Can you work these out from the model? Positions are in its coordinate system, mm. A direction names the side the tool comes from. Give positions to 0.01 mm unless a question says otherwise; leave off trailing zeros. Loops run counter-clockwise (first coordinate to the right, second up) from the corner with the lowest first, then second, coordinate; pieces in that order, holes last. Notation, with made-up numbers: (-15, 69) - (5, 69) arc R30 ccw to (5, 108) - close; hole circle Ø3 at (21.5, 85.25). An arc over 180 degrees is marked (long way). Answer as a JSON object with one key per item and string values. Group by question number.
Item 1: Suppose I cut it at B-B on z = -644.5. Write out the boundary of the cut face in (x, y).
Item 2: Thinking about a two-plate mould opening in Z: for faces 4 (the flat face through (646, 61, -711.2)), 5 (the flat face through (-650, 147, -685.8)), 6 (the flat face through (646, 132, -685.8)), 7 (the flat face through (646, -196.151, -698)), which applies, pulls with the +Z half, pulls with the -Z half, needs draft (parallel to the pull), parting line crosses it, or undercut?
Item 3: Suppose I cut it at A-A on y = 291. Write out the boundary of the cut face in (x, z).
Item 4: Please list where these lines run through material, in increasing order: L1, parallel to Y at x = 130.5, z = -12; L2, parallel to Z at x = -587, y = -171.5; L3, parallel to X at y = -108, z = -228.5.
Item 5: Which directions (+Z, -Z, +X, -X, +Y, -Y) give clear straight access to the entire face, cutting with the end or side of a thin tool? Please do faces 1 (the flat face through (646, -158, -685.8)), 2 (the flat face through (-650, -28.704, -357)), 3 (the flat face through (-650, 326.896, -698)).
Item 6: Will these pins go through, and if not, where does the flat tip stop? pin 1 (15 mm diameter, centred on x = -637, z = -520, fed in from +Y); pin 2 (2 mm diameter, centred on x = -191.5, z = -274.5, fed in from +Y); pin 3 (12.5 mm diameter, centred on x = -640.5, z = -697.5, fed in from -Y).
Item 7: Suppose I cut it at C-C on x = -510.5. Write out the boundary of the cut face in (y, z).
Item 8: Suppose I cut it at D-D on y = 100.5. Write out the boundary of the cut face in (x, z), and give its area (3 significant figures).
from build123d import *

# Parameters (mm, degrees)
F0_W           = 1346.2
F0_H           = 685.8
F1_DEPTH       = 25.4
F4_DEPTH       = 38.1
F2_W           = 50.8
F2_H           = 76.2
F5_DEPTH       = 685.8
F7_W           = 50.8
F7_H           = 25.4
F8_DEPTH       = 76.2
F8_DEPTH_BACK  = 431.8
F9_W           = 1244.6
F9_H           = 304.8
F10_DEPTH      = 25.4
F6_W           = 50.8
F6_H           = 25.4
F11_DEPTH      = 431.8
F11_DEPTH_BACK = 76.2


with BuildPart() as f1:
    # F0 (on Top) → F1 (new body)
    with BuildSketch(Plane.XY):
        with Locations((-1.6667507589, -3.4339692544)):
            Rectangle(F0_W, F0_H)
    extrude(amount=F1_DEPTH)

    # F3 (on face) → F4 (join)
    with BuildSketch(Plane(origin=(0, 0, 0), x_dir=(1, 0, 0), z_dir=(0, 0, -1))):
        Polygon((-674.7667507589, -254.2923092842), (671.4332492411, -254.2923092842), (671.4332492411, 35.8601883054), (-623.9667507589, 35.8601883054), (-623.9667507589, 28.7036430091), (-674.7667507589, 28.7036430091), align=None)
    extrude(amount=F4_DEPTH)

    # F2 (on face) → F5 (join)
    with BuildSketch(Plane(origin=(0, 0, 0), x_dir=(1, 0, 0), z_dir=(0, 0, -1))):
        with Locations((646.0332492411, 81.8509380281)):
            Rectangle(F2_W, F2_H)
        with Locations((-649.3667507589, 66.8036430091)):
            Rectangle(F2_W, F2_H)
    extrude(amount=F5_DEPTH)

    # F7 (on face) → F8 (join, two sides)
    with BuildSketch(Plane.XZ.offset(104.9036430091)) as f8_sk:
        with Locations((-649.3667507589, -698.5)):
            Rectangle(F7_W, F7_H)
    extrude(amount=F8_DEPTH)
    extrude(f8_sk.sketch, amount=-F8_DEPTH_BACK)

    # F9 (on face) → F10 (join)
    with BuildSketch(Plane.XZ.offset(104.9036430091)):
        with Locations((-1.6667507589, -152.4)):
            Rectangle(F9_W, F9_H)
    extrude(amount=-F10_DEPTH)

    # F6 (on face) → F11 (join, two sides)
    with BuildSketch(Plane.XZ.offset(119.9509380281)) as f11_sk:
        with Locations((646.0332492411, -698.5)):
            Rectangle(F6_W, F6_H)
    extrude(amount=-F11_DEPTH)
    extrude(f11_sk.sketch, amount=F11_DEPTH_BACK)


solid = f1.part
Worked out:
{
 "1": {"outline": "(-674.77, -104.9) - (-623.97, -104.9) - (-623.97, -28.7) - (-674.77, -28.7) - close; (620.63, -119.95) - (671.43, -119.95) - (671.43, -43.75) - (620.63, -43.75) - close"},
 "2": {"face 4": "pulls with the -Z half", "face 5": "undercut", "face 6": "undercut", "face 7": "needs draft"},
 "3": {"outline": "(-674.77, -711.2) - (-623.97, -711.2) - (-623.97, -685.8) - (-674.77, -685.8) - close; (-674.77, 0) - (671.43, 0) - (671.43, 25.4) - (-674.77, 25.4) - close; (620.63, -711.2) - (671.43, -711.2) - (671.43, -685.8) - (620.63, -685.8) - close"},
 "4": {"L1": "y = -104.9 to -79.5, -35.86 to 254.29", "L2": "z = 0 to 25.4", "L3": "x = 620.63 to 671.43"},
 "5": {"face 1": "+X, -X, -Y", "face 2": "+X, -X, +Y", "face 3": "-Z, +X, -X, +Y"},
 "6": {"pin 1": "stops at y = -28.7", "pin 2": "stops at y = -79.5", "pin 3": "stops at y = -181.1"},
 "7": {"outline": "(-346.33, 0) - (-104.9, 0) - (-104.9, -304.8) - (-79.5, -304.8) - (-79.5, 0) - (-35.86, 0) - (-35.86, -38.1) - (254.29, -38.1) - (254.29, 0) - (339.47, 0) - (339.47, 25.4) - (-346.33, 25.4) - close"},
 "8": {"outline": "(-674.77, -711.2) - (-623.97, -711.2) - (-623.97, -685.8) - (-674.77, -685.8) - close; (-674.77, -38.1) - (671.43, -38.1) - (671.43, 25.4) - (-674.77, 25.4) - close; (620.63, -711.2) - (671.43, -711.2) - (671.43, -685.8) - (620.63, -685.8) - close", "area": "88,100 mm2"}
}
